```python
from build123d import *

# Parameters (mm, degrees)
SKETCH_1_W          = 50
SKETCH_1_H          = 26
SKETCH_1_R          = 8.1
EXTRUDE_1_DEPTH     = 14
SKETCH_2_R          = 1.35
CUT_EXTRUDE_1_DEPTH = 5
SKETCH_3_W          = 12
SKETCH_3_H          = 4
CUT_EXTRUDE_2_DEPTH = 4
CHAMFER_1_SIZE      = 1
FILLET_1_R          = 2
CHAMFER_2_SIZE      = 1


with BuildPart() as part:
    # 草图1 → 凸台-拉伸1 (new body)
    with BuildSketch(Plane.XY):
        with Locations((0, 2)):
            Rectangle(SKETCH_1_W, SKETCH_1_H)
        with Locations((13, 0)):
            Circle(SKETCH_1_R, mode=Mode.SUBTRACT)
        with Locations((-13, 0)):
            Circle(SKETCH_1_R, mode=Mode.SUBTRACT)
    extrude(amount=EXTRUDE_1_DEPTH)

    # 草图2 → 切除-拉伸1 (cut)
    with BuildSketch(Plane(origin=(0, 15, 0), x_dir=(1, 0, 0), z_dir=(0, 1, 0))):
        with Locations(Location((-17.5, -10, 0), (0, 0, 270))):
            Circle(SKETCH_2_R)
        with Locations(Location((17.5, -10, 0), (0, 0, 270))):
            Circle(SKETCH_2_R)
    extrude(amount=-CUT_EXTRUDE_1_DEPTH, mode=Mode.SUBTRACT)

    # 草图3 → 切除-拉伸2 (cut)
    with BuildSketch(Plane(origin=(0, 0, 0), x_dir=(-1, 0, 0), z_dir=(0, 0, -1))):
        with Locations((0, 9)):
            Rectangle(SKETCH_3_W, SKETCH_3_H)
        with BuildLine():
            Line((-6, -11), (6, -11))
            Line((6, -11), (6, -7))
            ThreePointArc((6, -7), (5.707106781, -6.292893219), (5, -6))
            Line((5, -6), (-5, -6))
            ThreePointArc((-5, -6), (-5.707106781, -6.292893219), (-6, -7))
            Line((-6, -7), (-6, -11))
        make_face()
    extrude(amount=-CUT_EXTRUDE_2_DEPTH, mode=Mode.SUBTRACT)

    # 倒角1
    chamfer_1_edges = [part.edges().sort_by_distance(p)[0] for p in [
        (-21.1, 0, 14),
        (4.9, 0, 14),
    ]]
    chamfer(chamfer_1_edges, length=CHAMFER_1_SIZE)

    # 圆角1
    fillet_1_edges = [part.edges().sort_by_distance(p)[0] for p in [
        (-25, 15, 7),
        (25, 15, 7),
        (25, -11, 7),
        (-25, -11, 7),
    ]]
    fillet(fillet_1_edges, radius=FILLET_1_R)

    # 倒角2
    chamfer_2_edges = [part.edges().sort_by_distance(p)[0] for p in [
        (-25, 2, 14),
        (0, 15, 14),
        (0, -11, 14),
        (25, 2, 14),
        (-24.414213562, -10.414213562, 14),
        (24.414213562, -10.414213562, 14),
        (24.414213562, 14.414213562, 14),
        (-24.414213562, 14.414213562, 14),
    ]]
    chamfer(chamfer_2_edges, length=CHAMFER_2_SIZE)


solid = part.part
```
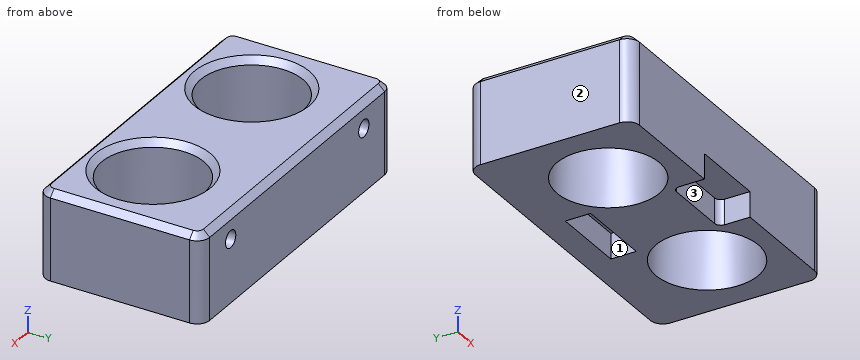
Could you check a few things on this model? Use its own coordinates, in mm. Face numbers are marked on the shaded views. A direction names the side the tool comes from. Round coordinates to 2 decimals unless told otherwise and drop trailing zeros. Loops run counter-clockwise (first coordinate to the right, second up) from the corner with the lowest first, then second, coordinate; pieces in that order, holes last. Notation, with made-up numbers: (-30.75, 65) - (2.25, 65) arc R18 cw to (2.25, 81) - close; hole circle Ø7 at (9.5, 0.5). An arc over 180 degrees is marked (long way). Answer in a Markdown table with one row per item. Add a question column.
(1) If we section it at B-B (x = 13): Please give me the cut outline in (y, z).
(2) If we section it at D-D (x = -1.5): Please give me the cut outline in (y, z), plus the area to 3 significant figures.
(3) If we section it at A-A (y = 0): Please give me the cut outline in (x, z).
(4) If we section it at C-C (z = 6.75): Please give me the cut outline in (x, y), plus the area to 3 significant figures.
(5) I'm going to push flat-ended pins straight in: pin 1 (1 mm diameter, centred on x = 4.5, y = 1, fed in from +Z); pin 2 (1.5 mm diameter, centred on x = 6.5, y = -6.5, fed in from -Z); pin 3 (4 mm diameter, centred on x = 2.5, y = -9.5, fed in from -Z). Where does each tip first touch, or does it pass through?
(6) I need wall thicknesses on line 1 along X through (y, z) = (12.85, 10); line 2 along Y through (x, z) = (-13, 10); line 3 along X through (y, z) = (13.7, 10). Which ranges of each line are inside material? Lowest first, please.
(7) For the marked faces 1, 2 and 3, which set-ups out of +Z, -Z, +X, -X, +Y, -Y let a thin tool reach every point of the face, with its end or its side?
Model answer:
| question | item | result |
|---|---|---|
| 1 | outline | (-11, 0) - (-8.1, 0) - (-8.1, 13) - (-9.1, 14) - (-10, 14) - (-11, 13) - close; (8.1, 0) - (15, 0) - (15, 13) - (14, 14) - (9.1, 14) - (8.1, 13) - close |
| 2 | outline | (-11, 4) - (-6, 4) - (-6, 0) - (7, 0) - (7, 4) - (11, 4) - (11, 0) - (15, 0) - (15, 13) - (14, 14) - (-10, 14) - (-11, 13) - close |
| 2 | area | 327 mm² |
| 3 | outline | (-25, 0) - (-21.1, 0) - (-21.1, 13) - (-22.1, 14) - (-24, 14) - (-25, 13) - close; (-4.9, 0) - (4.9, 0) - (4.9, 13) - (3.9, 14) - (-3.9, 14) - (-4.9, 13) - close; (21.1, 0) - (25, 0) - (25, 13) - (24, 14) - (22.1, 14) - (21.1, 13) - close |
| 4 | outline | (-25, -9) arc R2 ccw to (-23, -11) - (23, -11) arc R2 ccw to (25, -9) - (25, 13) arc R2 ccw to (23, 15) - (-23, 15) arc R2 ccw to (-25, 13) - close; hole circle Ø16.2 at (-13, 0); hole circle Ø16.2 at (13, 0) |
| 4 | area | 884 mm² |
| 5 | pin 1 | stops at z = 13.96 |
| 5 | pin 2 | stops at z = 0 |
| 5 | pin 3 | stops at z = 4 |
| 6 | line 1 | x = -25 to -18.85, -16.15 to 16.15, 18.85 to 25 |
| 6 | line 2 | y = -11 to -8.1, 8.1 to 15 |
| 6 | line 3 | x = -24.87 to -18.85, -16.15 to 16.15, 18.85 to 24.87 |
| 7 | face 1 | -Z |
| 7 | face 2 | +Z, -Z, -X, +Y, -Y |
| 7 | face 3 | -Z, -Y |
